from build123d import *

# Parameters (mm, degrees)
EXTRUDE1_DEPTH  = 180
SKETCH6_R       = 0.5
EXTRUDE2_DEPTH  = 181.103442499
LPATTERN1_COUNT = 11
LPATTERN1_PITCH = 15


with BuildPart() as part:
    # Sketch1 → Extrude1 (new body)
    with BuildSketch(Plane(origin=(0, 0, 0), x_dir=(0, 0, -1), z_dir=(1, 0, 0))):
        with BuildLine():
            Line((-3.5, 0.5), (-3, 0))
            Line((-3, 0), (3, 0))
            Line((3, 0), (3.5, 0.5))
            Line((3.5, 0.5), (3.5, 2.465153077))
            ThreePointArc((3.5, 2.465153077), (3.211148341, 2.591798371), (2.999904622, 2.826))
            Line((2.999904622, 2.826), (2.572, 2.90145113))
            ThreePointArc((2.572, 2.90145113), (2.501845147, 2.968757157), (2.45, 3.051))
            Line((2.45, 3.051), (2.45, 3.349))
            ThreePointArc((2.45, 3.349), (2.501845147, 3.431242843), (2.572, 3.49854887))
            Line((2.572, 3.49854887), (2.999904622, 3.574))
            ThreePointArc((2.999904622, 3.574), (3.211148341, 3.808201629), (3.5, 3.934846923))
            Line((3.5, 3.934846923), (3.5, 4.6))
            ThreePointArc((3.5, 4.6), (3.382052634, 4.824039475), (3.2, 5))
            Line((3.2, 5), (-3.2, 5))
            ThreePointArc((-3.2, 5), (-3.382052634, 4.824039475), (-3.5, 4.6))
            Line((-3.5, 4.6), (-3.5, 3.934846923))
            ThreePointArc((-3.5, 3.934846923), (-3.211148341, 3.808201629), (-2.999904622, 3.574))
            Line((-2.999904622, 3.574), (-2.572, 3.49854887))
            ThreePointArc((-2.572, 3.49854887), (-2.501845147, 3.431242843), (-2.45, 3.349))
            Line((-2.45, 3.349), (-2.45, 3.051))
            ThreePointArc((-2.45, 3.051), (-2.501845147, 2.968757157), (-2.572, 2.90145113))
            Line((-2.572, 2.90145113), (-2.999904622, 2.826))
            ThreePointArc((-2.999904622, 2.826), (-3.211148341, 2.591798371), (-3.5, 2.465153077))
            Line((-3.5, 2.465153077), (-3.5, 0.5))
        make_face()
    extrude(amount=EXTRUDE1_DEPTH)

    # Sketch2 → Cut-Revolve1 (revolve, cut)
    with BuildSketch(Plane(origin=(0, 0, 0), x_dir=(-1, 0, 0), z_dir=(0, 0, -1)), mode=Mode.PRIVATE) as cut_revolve1_sk:
        Polygon((-7.5, 5), (-5.4, 5), (-5.4, 2.7), (-6.3, 2.7), (-6.3, 0.2), (-6.1, 0), (-7.5, 0), align=None)
    revolve(cut_revolve1_sk.sketch.rotate(Axis((7.5, 0, 0), (0, 1, 0)), 90), axis=Axis((7.5, 0, 0), (0, 1, 0)), mode=Mode.SUBTRACT)

    # Sketch3 → Cut-Revolve2 (revolve, cut)
    with BuildSketch(Plane(origin=(45, 0, 0), x_dir=(-1, 0, 0), z_dir=(0, 0, -1)), mode=Mode.PRIVATE) as cut_revolve2_sk:
        Polygon((-127.5, 5), (-125.4, 5), (-125.4, 2.7), (-126.3, 2.7), (-126.3, 0.2), (-126.1, 0), (-127.5, 0), align=None)
    cut_revolve2 = revolve(cut_revolve2_sk.sketch.rotate(Axis((172.5, 0, 0), (0, 1, 0)), 90), axis=Axis((172.5, 0, 0), (0, 1, 0)), mode=Mode.SUBTRACT)

    # Sketch6 → Extrude2 (cut, through all)
    with BuildSketch(Plane(origin=(0, 0, 0), x_dir=(0, 0, -1), z_dir=(1, 0, 0))):
        with Locations((1.5, -0.3)):
            Circle(SKETCH6_R)
    extrude(amount=EXTRUDE2_DEPTH, mode=Mode.SUBTRACT)

    # LPattern1: Cut-Revolve2 ×11
    with Locations(*[(-i * LPATTERN1_PITCH, 0, 0) for i in range(1, LPATTERN1_COUNT)]):
        add(cut_revolve2, mode=Mode.SUBTRACT)


solid = part.part
Geometry: final body of the model. Coordinates: model frame, mm. A direction names the side the tool comes from. Coordinates: 2 decimals unless noted, no trailing zeros. One line per item, written item: value. Start each with the question number.
1) Draft query along X for faces 1 (the flat face through (180, 3, 0)), 2 (the flat face through (111, 2.7, 0)), 3 (the flat face through (0, 3, 0)). Return one class per face: released by +X, released by -X, zero draft, split by the parting line, or undercut.
2) Cut plane A-A (z = 0). Count the separate pieces of the cut face and the enclosed holes in it, then the cut area to 3 significant figures.
3) Reachability of faces 4 (the flat face through (96, 2.7, 0)), 5 (the flat face through (89, 5, 0)) from +Z, -Z, +X, -X, +Y, -Y: full face, straight path, thin tool, end or side. Return the list, or none.
4) Material intervals for L1, parallel to Y at x = 37, z = 2.75; L2, parallel to Y at x = 45, z = -3; L3, parallel to Y at x = 24.5, z = -0.5, sorted ascending. Write a range as from..to.
5) Pin query (flat end, axial travel): P1, Ø1.3, axis at x = 51.5, z = 0.5, coming from the +Y side; P2, Ø2.5, axis at x = 7.5, z = 0, coming from the -Y side; P3, Ø1.3, axis at x = 67.5, z = 0, coming from the +Y side. Return the tip coordinate at first contact, or that it passes through.
Evaluation:
1. face 1: released by +X
1. face 2: undercut
1. face 3: released by -X
2. separate pieces: 13
2. enclosed holes: 0
2. area: 706 mm^2
3. face 4: +Y
3. face 5: +Z, -Z, +X, -X, +Y
4. L1: 0..2.87, 3.53..5
4. L2: 0..2.83, 3.57..5
4. L3: 0..2.7
5. P1: y = 2.7
5. P2: y = 0.15
5. P3: through
